Check sheet for the modelled part. Datum: model origin and axes. Units: mm. A direction names the side the tool comes from. Coordinates: 2 decimals unless noted, no trailing zeros. Loops run counter-clockwise (first coordinate to the right, second up) from the corner with the lowest first, then second, coordinate; pieces in that order, holes last. Notation, with made-up numbers: (2, -34) - (56, -34) arc R12 cw to (56, -11) - close; hole circle Ø1 at (-19.5, 11). An arc over 180 degrees is marked (long way). Write each question's results on one line, items separated by ' | '. Start each with the question number.
1. Cross-section at B-B (z = -11.75). Record the cut outline in (x, y), and give its area (3 significant figures).
2. Draft check along X on faces 1 (the face through (0, 18, -15)), 2 (the face through (0, 0, -7.5)), 3 (the face through (7, -18, -6.6)), 4 (the face through (-4.769, 21.477, -1.521)). Enter one of: released by +X, released by -X, zero draft, split by the parting line, or undercut.
3. Thickness scan on line 1 (Z direction, x = 10, y = 16.5); line 2 (X direction, y = 0, z = -17.5); line 3 (Z direction, x = -18, y = 0). Record the ranges inside material, lowest first. Write a range as [from, to].
4. Tool access check on faces 5 (the face through (13.856, 5.745, -13.662)), 6 (the face through (20.32, 8.43, -13.39)), 7 (the face through (-7, -18, -3)). Record the directions out of +Z, -Z, +X, -X, +Y, -Y that give a thin tool (end or side, any length) a straight path to the whole face; none if there is none.
5. Cross-section at D-D (x = -1). Record the cut outline in (y, z).
6. Cross-section at A-A (y = 0). Record the cut outline in (x, z).
7. Gauge pin test, flat ends, axial feed: P1, Ø13, axis at x = -5.5, y = -4, coming from the -Z side; P2, Ø5, axis at x = -3, z = -17, coming from the +Y side; P3, Ø3, axis at y = 8, z = -10.5, coming from the -X side; P4, Ø8, axis at y = 0, z = -12.5, coming from the -X side. Record the tip position at first contact, or that the pin passes through.
8. Cross-section at C-C (x = -18). Record the cut outline in (y, z), and give its area (3 significant figures).
```python
from build123d import *

# Parameters (mm, degrees)
CORTE_EXTRUS_O1_REACH      = 55.104
CORTE_EXTRUS_O1_END_RADIUS = 15
ESBO_O3_R                  = 2.5
PADR_OCIRCULAR1_COUNT      = 4


with BuildPart() as part:
    # Esbo_o1 → Revolu_o1 (revolve)
    with BuildSketch(Plane(origin=(0, 0, 0), x_dir=(1, 0, 0), z_dir=(0, 1, 0)), mode=Mode.PRIVATE) as revolu_o1_sk:
        Polygon((0, 0), (-22, 0), (-22, 3), (-19, 3), (-19, 6.6), (-22, 6.6), (-22, 20), (-15, 20), (-15, 7.5), (0, 7.5), align=None)
    revolve(revolu_o1_sk.sketch.rotate(Axis((0, 0, 0), (0, 0, -1)), 180), axis=Axis((0, 0, 0), (0, 0, -1)))

    # Corte-extrus_o1: up to this cylinder (the profile starts outside it)
    corte_extrus_o1_end = Plane(origin=(0, 0, -12.5), z_dir=(0, 0, 1)) * Cylinder(CORTE_EXTRUS_O1_END_RADIUS, 141.208, mode=Mode.PRIVATE)
    # Esbo_o3 → Corte-extrus_o1 (cut, up to the surface)
    with BuildSketch(Plane.ZY.offset(22), mode=Mode.PRIVATE) as corte_extrus_o1_sk1:
        with Locations((-12.5, 0)):
            Circle(ESBO_O3_R)
    corte_extrus_o1_tool1 = extrude(corte_extrus_o1_sk1.sketch, amount=-CORTE_EXTRUS_O1_REACH, mode=Mode.PRIVATE) - corte_extrus_o1_end
    corte_extrus_o1 = corte_extrus_o1_tool1.solids().sort_by_distance((-22, 0, -12.5))[0]
    add(corte_extrus_o1, mode=Mode.SUBTRACT)

    # Padr_oCircular1: Corte-extrus_o1 ×4 about axis
    padr_ocircular1_axis = Axis((0, 0, -20), (0, 0, 1))
    for i in range(1, PADR_OCIRCULAR1_COUNT):
        add(corte_extrus_o1.rotate(padr_ocircular1_axis, i * 360 / PADR_OCIRCULAR1_COUNT), mode=Mode.SUBTRACT)


solid = part.part
```
Established:
1) outline: (-21.87, -2.38) arc R22 ccw to (-2.38, -21.87) - (-2.38, -14.81) arc R15 cw to (-14.81, -2.38) - close; (-21.87, 2.38) - (-14.81, 2.38) arc R15 cw to (-2.38, 14.81) - (-2.38, 21.87) arc R22 ccw to start; (2.38, -21.87) arc R22 ccw to (21.87, -2.38) - (14.81, -2.38) arc R15 cw to (2.38, -14.81) - close; (2.38, 14.81) arc R15 cw to (14.81, 2.38) - (21.87, 2.38) arc R22 ccw to (2.38, 21.87) - close | area: 680 mm^2
2) face 1: undercut | face 2: undercut | face 3: zero draft | face 4: split by the parting line
3) line 1: [-20, -6.6], [-3, 0] | line 2: [-22, -15], [15, 22] | line 3: [-20, -15], [-10, 0]
4) face 5: -Z | face 6: +Z, -Z | face 7: none
5) outline: (-21.98, -20) - (-14.97, -20) - (-14.97, -14.79) - (-21.98, -14.79) - close; (-21.98, -10.21) - (-14.97, -10.21) - (-14.97, -7.5) - (14.97, -7.5) - (14.97, -10.21) - (21.98, -10.21) - (21.98, -6.6) - (18.97, -6.6) - (18.97, -3) - (21.98, -3) - (21.98, 0) - (-21.98, 0) - (-21.98, -3) - (-18.97, -3) - (-18.97, -6.6) - (-21.98, -6.6) - close; (14.97, -20) - (21.98, -20) - (21.98, -14.79) - (14.97, -14.79) - close
6) outline: (-22, -20) - (-15, -20) - (-15, -15) - (-22, -15) - close; (-22, -10) - (-15, -10) - (-15, -7.5) - (15, -7.5) - (15, -10) - (22, -10) - (22, -6.6) - (19, -6.6) - (19, -3) - (22, -3) - (22, 0) - (-22, 0) - (-22, -3) - (-19, -3) - (-19, -6.6) - (-22, -6.6) - close; (15, -20) - (22, -20) - (22, -15) - (15, -15) - close
7) P1: z = -7.5 | P2: y = 21.99 | P3: x = -21.02 | P4: x = -22
8) outline: (-12.65, -20) - (12.65, -20) - (12.65, -6.6) - (6.08, -6.6) - (6.08, -3) - (12.65, -3) - (12.65, 0) - (-12.65, 0) - (-12.65, -3) - (-6.08, -3) - (-6.08, -6.6) - (-12.65, -6.6) - close; hole circle Ø5 at (0, -12.5) | area: 439 mm^2
